from build123d import *

# Parameters (mm, degrees)
F1_DEPTH = 3.0988
F0_W     = 3.175
F0_H     = 1.778
F2_DEPTH = 3.0988
F3_R     = 1.651


with BuildPart() as f1:
    # F0 (on Top) → F1 (new body)
    with BuildSketch(Plane.XY):
        with BuildLine():
            ThreePointArc((14.306537, -9.789921), (0, 17.3355), (-14.306537, -9.789921))
            Line((-14.306537, -9.789921), (-10.414, -28.437995))
            ThreePointArc((-10.414, -28.437995), (0, -35.8775), (10.414, -28.437995))
            Line((10.414, -28.437995), (14.306537, -9.789921))
        make_face()
        with BuildLine():
            Line((1.5875, -16.8275), (-1.5875, -16.8275))
            Line((-1.5875, -16.8275), (-1.5875, -21.0185))
            Line((-1.5875, -21.0185), (-11.43, -9.789921))
            ThreePointArc((-11.43, -9.789921), (0, 15.0495), (11.43, -9.789921))
            Line((11.43, -9.789921), (1.5875, -21.0185))
            Line((1.5875, -21.0185), (1.5875, -16.8275))
        make_face(mode=Mode.SUBTRACT)
    extrude(amount=F1_DEPTH)

    # F0 (on Top) → F2 (join)
    with BuildSketch(Plane.XY):
        with Locations((0, -15.9385)):
            Rectangle(F0_W, F0_H)
    extrude(amount=F2_DEPTH)

    # F3
    f3_edges = [f1.edges().sort_by_distance(p)[0] for p in [
        (-1.5875, -21.0185, 1.5494),
        (1.5875, -21.0185, 1.5494),
    ]]
    fillet(f3_edges, radius=F3_R)


solid = f1.part
Part model, mm, in its own coordinate system. A direction names the side the tool comes from. Coordinates: 2 decimals unless noted, no trailing zeros. Write each loop counter-clockwise with the first axis right and the second up, starting at its lowest first coordinate (ties: lowest second). Pieces come first, ordered by that corner, then holes. Notation, with made-up numbers: (51.25, 3.5) - (97.25, 3.5) arc R16 cw to (97.25, 28.5) - close; hole circle Ø5 at (37, 24.5). An arc over 180 degrees is marked (long way). Put each result on its own line as item: value.
1. Band-saw the part on B-B (x = 0). Write the cut outline in (y, z), then the cut area to 3 significant figures.
Final values:
outline: (-35.88, 0) - (-15.05, 0) - (-15.05, 3.1) - (-35.88, 3.1) - close; (15.05, 0) - (17.34, 0) - (17.34, 3.1) - (15.05, 3.1) - close
area: 71.6 mm²
2. Band-saw the part on A-A (y = 0). Write the cut outline in (x, z).
Final values:
outline: (-17.34, 0) - (-15.05, 0) - (-15.05, 3.1) - (-17.34, 3.1) - close; (15.05, 0) - (17.34, 0) - (17.34, 3.1) - (15.05, 3.1) - close
3. Probe line 1 along Y through (x, z) = (0, 1.3); line 2 along X through (y, z) = (0, 1.2); line 3 along X through (y, z) = (-15.5, 0.4). List the from-to ranges inside material, lowest first. Write a range as [from, to].
Final values:
line 1: y = [-35.88, -15.05], [15.05, 17.34]
line 2: x = [-17.34, -15.05], [15.05, 17.34]
line 3: x = [-13.11, -6.42], [-1.59, 1.59], [6.42, 13.11]
4. Band-saw the part on D-D (y = -29.5). Write the cut outline in (x, z).
Final values:
outline: (-9.99, 0) - (9.99, 0) - (9.99, 3.1) - (-9.99, 3.1) - close
5. Two-plate mould, pull along X, no slides. Class faces 1 (the cylindrical face through (2.631, -18.165, 1.571)), 2 (the cylindrical face through (-0.191, -35.876, 1.528)), 3 (the flat face through (1, -17, 0)): +X half, -X half, draft (parallel to the pull), parting line (faces both ways), or undercut.
Final values:
face 1: undercut
face 2: parting line
face 3: draft
6. Flat gauge pins, fed straight in: pin 1 Ø6 at (x, y) = (7.5, 7.5) entering from +Z; pin 2 Ø0.5 at (y, z) = (-16, 2) entering from +X; pin 3 Ø0.8 at (y, z) = (-15.5, 1.5) entering from -X; pin 4 Ø1.5 at (x, z) = (9.5, 1) entering from -Y. Where does each tip first touch, or does it go through?
Final values:
pin 1: passes through
pin 2: stops at x = 13.06
pin 3: stops at x = -13.2
pin 4: stops at y = -31.55
7. 3-axis set-ups, long thin cutter, end or side, ignore diameter. For faces 4 (the flat face through (-7.906, -13.81, 1.528)), 5 (the flat face through (12.333, -19.244, 1.528)): which of +Z, -Z, +X, -X, +Y, -Y reach the whole face in a straight line?
Final values:
face 4: +Z, -Z
face 5: +Z, -Z, +X, -Y
8. Band-saw the part on C-C (z = 0.85). Write the cut outline in (x, y).
Final values:
outline: (-14.31, -9.79) - (-10.41, -28.44) arc R11.01 ccw to (10.41, -28.44) - (14.31, -9.79) arc R17.34 ccw (long way) to start; hole (-11.43, -9.79) - (-4.48, -17.72) arc R1.65 ccw to (-1.59, -16.63) - (-1.59, -15.05) - (1.59, -15.05) - (1.59, -16.63) arc R1.65 ccw to (4.48, -17.72) - (11.43, -9.79) arc R15.05 ccw (long way) to start
